Check sheet for the drawn part. Datum: minimum x, y, z corner. Units: mm. A direction names the side the tool comes from. Coordinates: 2 decimals unless noted, no trailing zeros. Loops run counter-clockwise (first coordinate to the right, second up) from the corner with the lowest first, then second, coordinate; pieces in that order, holes last. Notation, with made-up numbers: (49, -11) - (65, -11) arc R18 cw to (65, 24) - close; hole circle Ø5 at (-7.5, -12.5). An arc over 180 degrees is marked (long way). Write item = value, one per line. Start each with the question number.
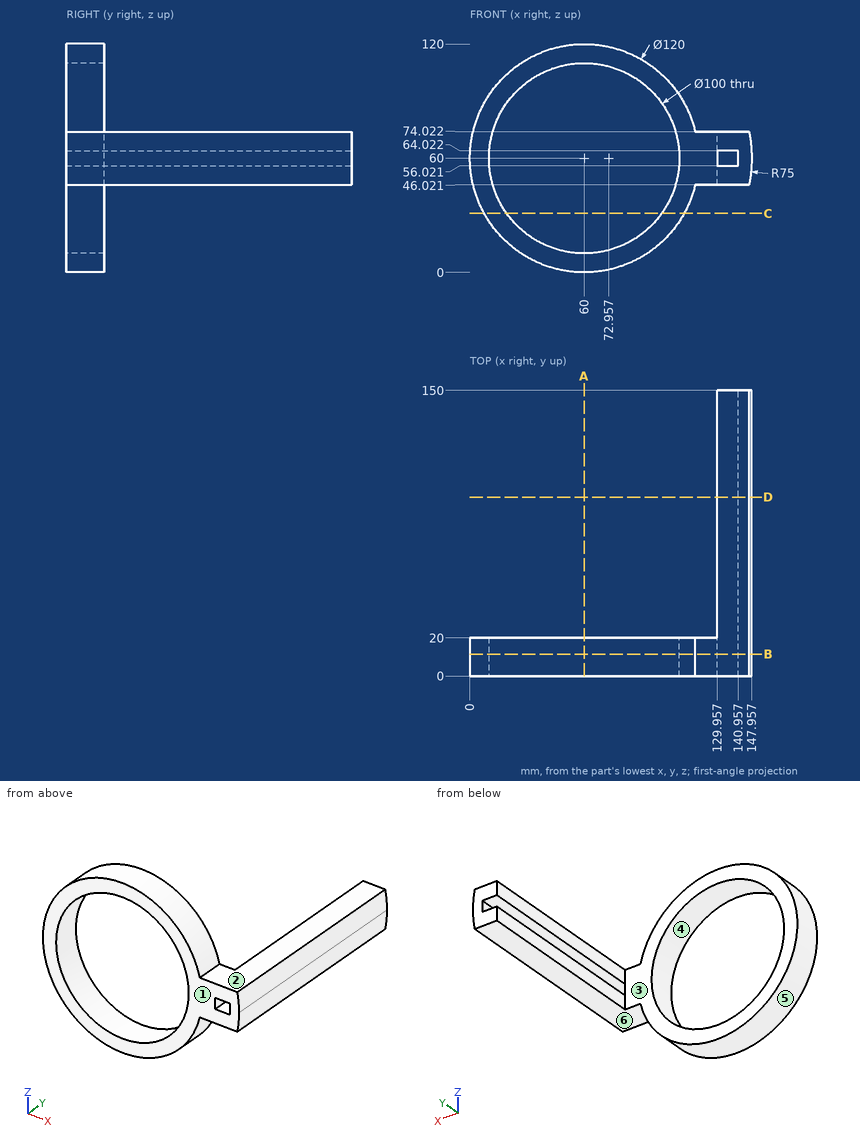
(1) Sectioned sample at A-A on x = 60. Enter the section's corners in (y, z).
(2) Depth check by flat-ended pin: pin 1 (8 mm diameter, centred on y = 56, z = 52.5, fed in from -X); pin 2 (3 mm diameter, centred on x = 122.5, z = 49, fed in from -Y); pin 3 (3.5 mm diameter, centred on x = 137.5, y = 38.5, fed in from +Z); pin 4 (6 mm diameter, centred on y = 103, z = 78.5, fed in from -X) (3 decimals). Enter the tip coordinate at first touch or a pass-through.
(3) Sectioned sample at D-D on y = 94. Enter the section's corners in (x, z), plus the area to 3 significant figures.
(4) Draft check along Z on the marked faces 4, 5 and 6. Enter one of: pulls with the +Z half, pulls with the -Z half, needs draft (parallel to the pull), parting line crosses it, or undercut.
(5) Sectioned sample at C-C on z = 31. Enter the section's corners in (x, y), plus the area to 3 significant figures.
(6) Scan lines: line 1 (X direction, y = 12.75, z = 60); line 2 (Z direction, x = 60, y = 5.5); line 3 (Z direction, x = 138, y = 82). Record each from-to range of solid material in increasing order.
(7) Tool access check on the marked faces 1, 2 and 3. Record the directions out of +Z, -Z, +X, -X, +Y, -Y that give a thin tool (end or side, any length) a straight path to the whole face; none if there is none.
(8) Sectioned sample at B-B on y = 11.5. Enter the section's corners in (x, z).
Working result:
q1.outline = (0, 0) - (20, 0) - (20, 10) - (0, 10) - close; (0, 110) - (20, 110) - (20, 120) - (0, 120) - close
q2.pin_1 = 129.96
q2.pin_2 = 0
q2.pin_3 = 74.02
q2.pin_4 = through
q3.outline = (129.96, 46.02) - (146.64, 46.02) arc R75 ccw to (146.63, 74.02) - (129.96, 74.02) - (129.96, 64.02) - (140.96, 64.02) - (140.96, 56.02) - (129.96, 56.02) - close
q3.area = 404 mm2
q4.face_4 = undercut
q4.face_5 = parting line crosses it
q4.face_6 = pulls with the -Z half
q5.outline = (7.47, 0) - (19.27, 0) - (19.27, 20) - (7.47, 20) - close; (100.73, 0) - (112.53, 0) - (112.53, 20) - (100.73, 20) - close
q5.area = 472 mm2
q6.line_1 = 0 to 10, 110 to 129.96, 140.96 to 147.96
q6.line_2 = 0 to 10, 110 to 120
q6.line_3 = 46.02 to 56.02, 64.02 to 74.02
q7.face_1 = +Z, -Z, +X, -X, -Y
q7.face_2 = +Z, +X, +Y, -Y
q7.face_3 = +Z, -Z, -X, +Y
q8.outline = (118.34, 74.02) arc R60 ccw (long way) to (118.35, 46.02) - (146.64, 46.02) arc R75 ccw to (146.63, 74.02) - close; hole circle Ø100 at (60, 60); hole (129.96, 56.02) - (140.96, 56.02) - (140.96, 64.02) - (129.96, 64.02) - close
